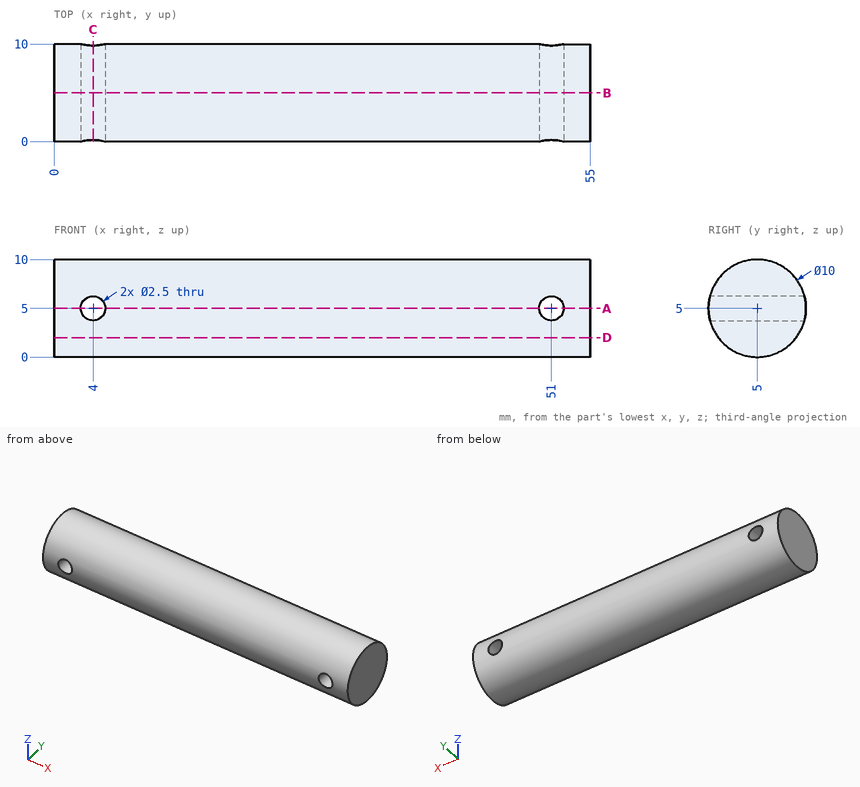
Part print with two shaded views. Sizes in mm from the minimum x, y, z corner. Round coordinates to 2 decimals unless told otherwise and drop trailing zeros. Order: outer loops, then holes, each group sorted by start corner. A loop starts at its lowest first (then second) coordinate and runs counter-clockwise, first axis right, second up. Notation, with made-up numbers: (63.5, 41.5) -> (100.5, 41.5) arc R15 cw to (100.5, 67.5) -> close; hole circle Ø1 at (51, -6). An arc over 180 degrees is marked (long way). Use one line per item in the form item = value.
Item 1: Cut at B-B, the plane y = 5. Write the cut outline in (x, z), and give its area (3 significant figures).
Returned:
outline = (0, 0) -> (55, 0) -> (55, 10) -> (0, 10) -> close; hole circle Ø2.5 at (4, 5); hole circle Ø2.5 at (51, 5)
area = 540 mm^2
Item 2: Cut at D-D, the plane z = 2. Write the cut outline in (x, y), and give its area (3 significant figures).
Returned:
outline = (0, 1) -> (55, 1) -> (55, 9) -> (0, 9) -> close
area = 440 mm^2
Item 3: Cut at C-C, the plane x = 4. Write the cut outline in (y, z).
Returned:
outline = (0.16, 3.75) arc R5 ccw to (9.84, 3.75) -> close; (0.16, 6.25) -> (9.84, 6.25) arc R5 ccw to start
Item 4: Flat gauge pins, fed straight in: pin 1 Ø4 at (x, y) = (22, 7.5) entering from +Z; pin 2 Ø5 at (x, z) = (17, 8) entering from -Y; pin 3 Ø5 at (x, y) = (47.5, 1.5) entering from -Z. Where does each tip first touch, or does it go through?
Returned:
pin_1 = 9.97
pin_2 = 0.03
pin_3 = 0.1
Item 5: Drill centre lines: line 1 (X direction, y = 6.5, z = 5); line 2 (X direction, y = 1.5, z = 6); line 3 (Z direction, x = 37.5, y = 4.75). Where is each one in solid material? Low to high.
Returned:
line_1 = 0 to 2.75, 5.25 to 49.75, 52.25 to 55
line_2 = 0 to 3.25, 4.75 to 50.25, 51.75 to 55
line_3 = 0.01 to 9.99
Item 6: Cut at A-A, the plane z = 5. Write the cut outline in (x, y).
Returned:
outline = (0, 0) -> (2.75, 0) -> (2.75, 10) -> (0, 10) -> close; (5.25, 0) -> (49.75, 0) -> (49.75, 10) -> (5.25, 10) -> close; (52.25, 0) -> (55, 0) -> (55, 10) -> (52.25, 10) -> close
